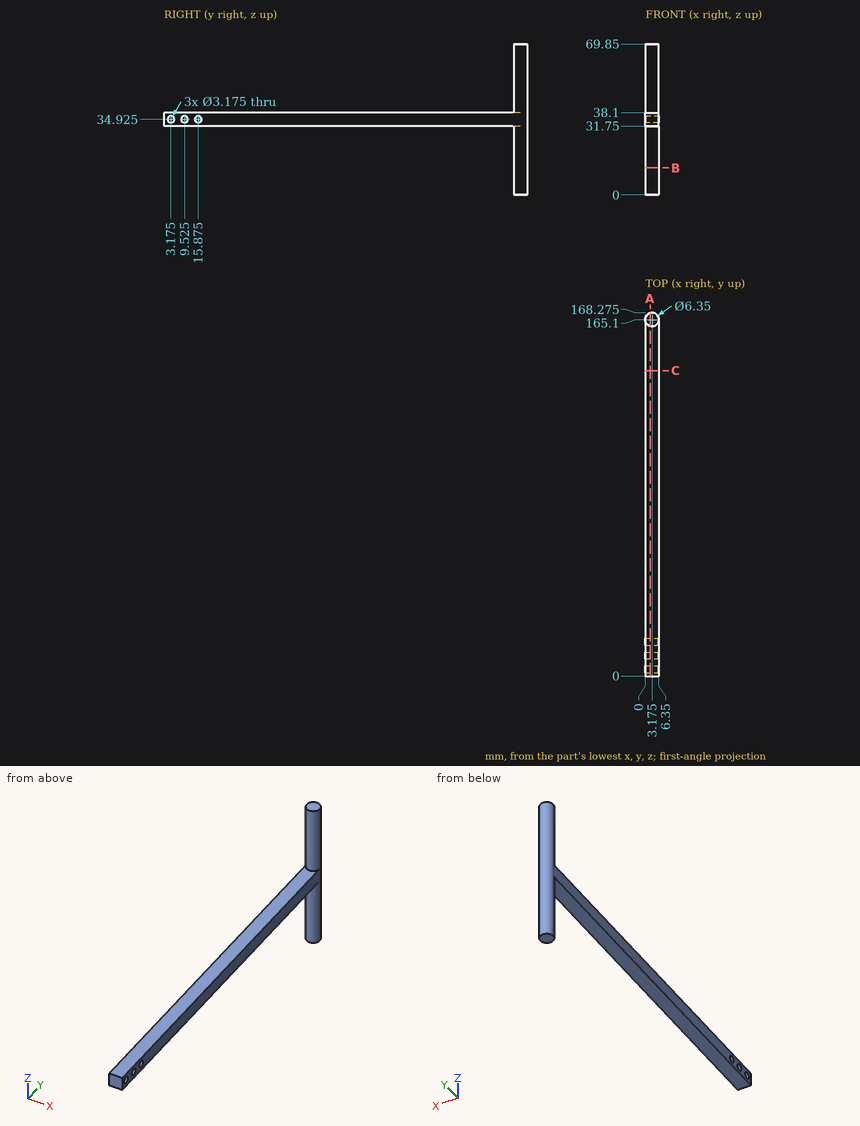
Here's the drawing with two shaded views (mm, measured from the low corner). I have some questions. Coordinates: 2 decimals unless noted, no trailing zeros. Write each loop counter-clockwise with the first axis right and the second up, starting at its lowest first coordinate (ties: lowest second). Pieces come first, ordered by that corner, then holes. Notation, with made-up numbers: (21, 89) -> (68, 89) arc R4 ccw to (68, 95) -> close; hole circle Ø6 at (-23.5, 84.5). An arc over 180 degrees is marked (long way). Use a Markdown table: item, result. Add a question column.
(1) If we section it at B-B, the plane z = 12.5: Write out the boundary of the cut face in (x, y) (3 decimals).
(2) If we section it at A-A, the plane x = 2.25: State how many separate pieces and enclosed holes the cut face has, and give its area (3 significant figures).
(3) If we section it at C-C, the plane y = 141.5: Write out the boundary of the cut face in (x, z).
(4) Please list where these lines run through material, in increasing order: line 1 (Z direction, x = 5.5, y = 144); line 2 (Y direction, x = 3.5, z = 54); line 3 (Y direction, x = 3.75, z = 35).
Outcome:
| question | item | result |
|---|---|---|
| 1 | outline | circle Ø6.35 at (3.175, 165.1) |
| 2 | separate pieces | 1 |
| 2 | enclosed holes | 3 |
| 2 | area | 1,430 mm^2 |
| 3 | outline | (0, 31.75) -> (6.35, 31.75) -> (6.35, 38.1) -> (0, 38.1) -> close |
| 4 | line 1 | z = 31.75 to 38.1 |
| 4 | line 2 | y = 161.94 to 168.26 |
| 4 | line 3 | y = 0 to 1.59, 4.76 to 7.94, 11.11 to 14.29, 17.46 to 168.22 |
